The model under review builds one solid part; all positions refer to its coordinate system, in mm. Face numbers are marked on the shaded views. A direction names the side the tool comes from. Coordinates: 2 decimals unless noted, no trailing zeros. Loops run counter-clockwise (first coordinate to the right, second up) from the corner with the lowest first, then second, coordinate; pieces in that order, holes last. Notation, with made-up numbers: M -32.75,47 L -24.75,47 A30 ccw -24.75,82 Z; hole C 40,-18 d2. An arc over 180 degrees is marked long. Return JSON: item names as keys, results as strings.
Autodesk Inventor part; units mm, degrees
ref_plane "YZ Plane" through (0, 0, 0) normal (1, 0, 0) x (0, 1, 0)
ref_plane "XZ Plane" through (0, 0, 0) normal (0, 1, 0) x (-1, 0, 0)
ref_plane "XY Plane" through (0, 0, 0) normal (0, 0, 1) x (1, 0, 0)
sketch "Sketch1" plane through (0, 0, 0) normal (0, 0, 1) x (1, 0, 0)
  circle A0 centre (0, 0) radius 3.81
  dimension "d0" = 7.62
extrude "Extrusion1" add sketch "Sketch1" along normal blind 5.08
sketch "Sketch2" plane through (0, 0, 5.08) normal (0, 0, 1) x (1, 0, 0)
  line L0 (1.2832, 2.2225) -> (2.5663, 0)
  line L1 (2.5663, 0) -> (1.2832, -2.2225)
  line L2 (1.2832, -2.2225) -> (-1.2832, -2.2225)
  line L3 (-1.2832, -2.2225) -> (-2.5663, 0)
  line L4 (-2.5663, 0) -> (-1.2832, 2.2225)
  line L5 (-1.2832, 2.2225) -> (1.2832, 2.2225)
  line L6 (0, 0) -> (0.4307, 0)
  dimension "d3" = 4.445
extrude "Extrusion2" cut sketch "Sketch2" against normal blind 2.54
sketch "Sketch3" plane through (0, 0, 0) normal (0, 0, -1) x (-1, 0, 0)
  circle A0 centre (0, 0) radius 2.0701
  dimension "d6" = 4.1402
extrude "Extrusion3" add sketch "Sketch3" along normal blind 39.37
properties part number "RobotArm Rivet2"
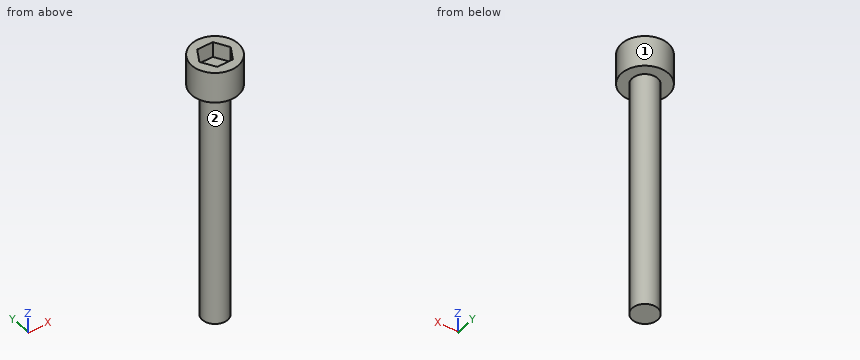
1. Insertion check: pin 1 Ø1.5 at (x, y) = (-2.5, -2.5) entering from -Z; pin 2 Ø4 at (y, z) = (0.5, -32.5) entering from -X; pin 3 Ø2 at (y, z) = (2, -1.5) entering from -X. Each pin has a flat end and moves straight along its axis. Give the tip position at first contact, or say it passes through.
Check values:
{"pin 1": "z = 0", "pin 2": "x = -2.07", "pin 3": "x = -1.81"}
2. Add section B-B on y = -0.75. Give the boundary of the cut face in (x, z).
Check values:
{"outline": "M -3.74,0 L -1.93,0 L -1.93,-39.37 L 1.93,-39.37 L 1.93,0 L 3.74,0 L 3.74,5.08 L 2.13,5.08 L 2.13,2.54 L -2.13,2.54 L -2.13,5.08 L -3.74,5.08 Z"}
3. Add section C-C on z = -33.5. Give the boundary of the cut face in (x, y).
Check values:
{"outline": "C 0,0 d4.14"}
4. Add section A-A on x = 0. Give the boundary of the cut face in (y, z), plus the area to 3 significant figures.
Check values:
{"outline": "M -3.81,0 L -2.07,0 L -2.07,-39.37 L 2.07,-39.37 L 2.07,0 L 3.81,0 L 3.81,5.08 L 2.22,5.08 L 2.22,2.54 L -2.22,2.54 L -2.22,5.08 L -3.81,5.08 Z", "area": "190 mm²"}
5. To check wall thickness, follow line 1 (Z direction, x = 1, y = 1.75); line 2 (Z direction, x = -1.25, y = 3.5); line 3 (X direction, y = 1.25, z = -11). State the ranges of each line that lie inside material, in increasing order.
Check values:
{"line 1": "-39.37 to 2.54", "line 2": "0 to 5.08", "line 3": "-1.65 to 1.65"}
6. Machinability: for the marked faces 1 and 2, which of the approach directions +Z, -Z, +X, -X, +Y, -Y give a long, thin tool a straight path to every point of the face, cutting with its end or side? Answer none if there is none.
Check values:
{"face 1": "+Z, -Z", "face 2": "-Z"}
7. Add section D-D on x = -3.25. Give the boundary of the cut face in (y, z), plus the area to 3 significant figures.
Check values:
{"outline": "M -1.99,0 L 1.99,0 L 1.99,5.08 L -1.99,5.08 Z", "area": "20.2 mm²"}
